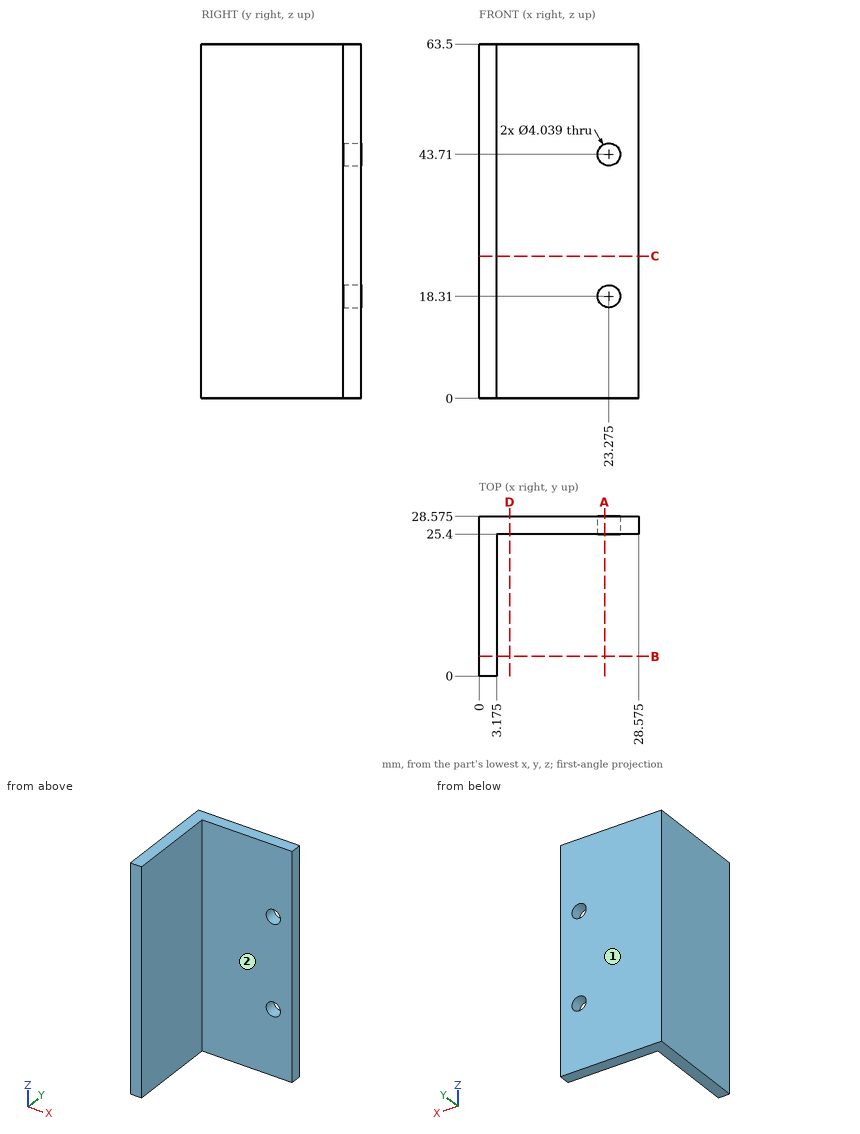
Design review of the part shown in the three views and the two pictorial views. Dimensions are in mm from the part's minimum x, y and z. A direction names the side the tool comes from. Round coordinates to 2 decimals unless told otherwise and drop trailing zeros. Write each loop counter-clockwise with the first axis right and the second up, starting at its lowest first coordinate (ties: lowest second). Pieces come first, ordered by that corner, then holes. Notation, with made-up numbers: (29, 3) -> (56, 3) arc R22 ccw to (56, 31) -> close; hole circle Ø4 at (1.5, 66). An arc over 180 degrees is marked (long way). One line per question, with ' | ' between items. Start each with the question number.
1) Machinability: for the marked faces 1 and 2, which of the approach directions +Z, -Z, +X, -X, +Y, -Y give a long, thin tool a straight path to every point of the face, cutting with its end or side? Answer none if there is none.
2) Add section C-C (z = 25.5). Write out the cut boundary in (x, y) (1 decimal), and give its area (3 significant figures).
3) Add section D-D (x = 5.5). Write out the cut boundary in (y, z) (1 decimal), and give its area (3 significant figures).
4) Wall thickness on line 1 along X through (y, z) = (18.25, 3) (1 decimal); line 2 along Y through (x, z) = (10, 13) (1 decimal): over which ranges is each line inside the solid? List them lowest first.
5) Add section B-B (y = 3.5). Write out the cut boundary in (x, z) (1 decimal), and give its area (3 significant figures).
6) Add section A-A (x = 22.5). Write out the cut boundary in (y, z) (1 decimal).
7) For pin 1 Ø6.5 at (x, z) = (23.28, 18.31) entering from -Y; pin 2 Ø8 at (y, z) = (6.5, 18) entering from +X (3 decimals); pin 3 Ø3 at (x, y) = (5, 14.5) entering from +Z, all flat-tipped, find the tip position at first contact; note any pin that passes through.
Reported:
1) face 1: +Z, -Z, +X, -X, +Y | face 2: +Z, -Z, +X, -Y
2) outline: (0, 0) -> (3.2, 0) -> (3.2, 25.4) -> (28.6, 25.4) -> (28.6, 28.6) -> (0, 28.6) -> close | area: 171 mm²
3) outline: (25.4, 0) -> (28.6, 0) -> (28.6, 63.5) -> (25.4, 63.5) -> close | area: 202 mm²
4) line 1: x = 0 to 3.2 | line 2: y = 25.4 to 28.6
5) outline: (0, 0) -> (3.2, 0) -> (3.2, 63.5) -> (0, 63.5) -> close | area: 202 mm²
6) outline: (25.4, 0) -> (28.6, 0) -> (28.6, 16.4) -> (25.4, 16.4) -> close; (25.4, 20.2) -> (28.6, 20.2) -> (28.6, 41.8) -> (25.4, 41.8) -> close; (25.4, 45.6) -> (28.6, 45.6) -> (28.6, 63.5) -> (25.4, 63.5) -> close
7) pin 1: stops at y = 25.4 | pin 2: stops at x = 3.175 | pin 3: passes through
